Autodesk Inventor part; units mm, degrees
ref_plane "YZ Plane" through (0, 0, 0) normal (1, 0, 0) x (0, 1, 0)
ref_plane "XZ Plane" through (0, 0, 0) normal (0, 1, 0) x (-1, 0, 0)
ref_plane "XY Plane" through (0, 0, 0) normal (0, 0, 1) x (1, 0, 0)
sketch "Esquisse1" plane through (0, 0, 0) normal (0, 0, 1) x (1, 0, 0)
  circle A0 centre (0, 0) radius 11
  circle A1 centre (0, 0) radius 8 construction
  line L0 (0, 0) -> (8, 0) construction
  circle A2 centre (8, 0) radius 1
  line L1 (0, 0) -> (0, 8) construction
  circle A3 centre (0, 8) radius 1
  line L2 (0, 0) -> (-8, 0) construction
  circle A4 centre (-8, 0) radius 1
  line L3 (0, 0) -> (0, -8) construction
  circle A5 centre (0, -8) radius 1
  dimension "d1" = 16
  dimension "d0" = 22
  dimension "d3" = 2
  dimension "d6" = 360
extrude "Extrusion1" add sketch "Esquisse1" along normal blind 5
sketch "Esquisse2" plane through (0, 0, 5) normal (0, 0, 1) x (1, 0, 0)
  circle A0 centre (0, 0) radius 11
  circle A1 centre (0, 0) radius 4
  dimension "d10" = 8
extrude "Extrusion2" add sketch "Esquisse2" along normal blind 40 contours A1
sketch "Esquisse3" plane through (0, 0, 0) normal (0, 0, -1) x (-1, 0, 0)
  circle A0 centre (0, 0) radius 11
  circle A1 centre (0, 0) radius 4
  dimension "d14" = 8
extrude "Extrusion3" cut sketch "Esquisse3" against normal blind 1.5 contours A1
fillet "Congé1" radius 3 1 edges at (-4, 0, 5)
properties part number "ax12tobase"
The model under review builds one solid part; all positions refer to its coordinate system, in mm. A direction names the side the tool comes from. Give positions to 0.01 mm unless a question says otherwise; leave off trailing zeros. Write each loop counter-clockwise with the first axis right and the second up, starting at its lowest first coordinate (ties: lowest second). Pieces come first, ordered by that corner, then holes. Notation, with made-up numbers: (84.25, -1.5) -> (96.25, -1.5) arc R25 ccw to (96.25, 15.5) -> close; hole circle Ø6 at (82, 73). An arc over 180 degrees is marked (long way). Answer in a Markdown table with one row per item.
1) For L1, parallel to Y at x = 0, z = 3.95; L2, parallel to Y at x = 0, z = 1.1; L3, parallel to Z at x = 9, y = -3.75, list the stretches that pass through material, from the lowest coordinate up. Write a range as [from, to].
Worked answers:
| item | result |
|---|---|
| L1 | [-11, -9], [-7, 7], [9, 11] |
| L2 | [-11, -9], [-7, -4], [4, 7], [9, 11] |
| L3 | [0, 5] |
2) Tool access review of faces 1 (the flat face through (0, 0, 1.5)), 2 (the cylindrical face through (-8.8, 0.6, 2.5)), 3 (the flat face through (7, -2, 5)): name each direction out of +Z, -Z, +X, -X, +Y, -Y from which nothing blocks a thin tool from reaching the whole face with its end or side.
Worked answers:
| item | result |
|---|---|
| face 1 | -Z |
| face 2 | +Z, -Z |
| face 3 | +Z |
3) Clearance check with flat-ended pins moving along their axes: P1, Ø3, axis at x = 0, y = -8, coming from the +Z side; P2, Ø12, axis at x = -2.5, z = 15.5, coming from the -Y side; P3, Ø5, axis at x = 6, z = 25, coming from the +Y side; P4, Ø1.2, axis at x = 8, y = 0, coming from the -Z side. State where each tip first meets the part, or that it passes through.
Worked answers:
| item | result |
|---|---|
| P1 | z = 5.04 |
| P2 | y = -4 |
| P3 | y = 1.94 |
| P4 | through |
4) Add section A-A on x = 0. Count the separate pieces of the cut face and the enclosed holes in it, plus the area to 3 significant figures.
Worked answers:
| item | result |
|---|---|
| separate pieces | 3 |
| enclosed holes | 0 |
| area | 402 mm² |
5) Mouldability with a two-part tool opening along Y and no side actions: class faces 4 (the cylindrical face through (0.867, -3.905, 0.74)), 5 (the cylindrical face through (7.2, 0.6, 2.5)), 6 (the flat face through (0, 0, 45)), 7 (the cylindrical face through (-0.867, 3.905, 26.241)) as +Y half, -Y half, draft (parallel to the pull), parting line (faces both ways), or undercut.
Worked answers:
| item | result |
|---|---|
| face 4 | undercut |
| face 5 | undercut |
| face 6 | draft |
| face 7 | parting line |
6) Add section C-C on y = -8. State the section outline as (x, z) points.
Worked answers:
| item | result |
|---|---|
| outline | (-7.55, 0) -> (-1, 0) -> (-1, 5) -> (-7.55, 5) -> close; (1, 0) -> (7.55, 0) -> (7.55, 5) -> (1, 5) -> close |
